Read the model definition and answer for the solid it produces. Units are mm, in the model's axes. A direction names the side the tool comes from. Give positions to 0.01 mm unless a question says otherwise; leave off trailing zeros. Order: outer loops, then holes, each group sorted by start corner. A loop starts at its lowest first (then second) coordinate and runs counter-clockwise, first axis right, second up. Notation, with made-up numbers: (58, -29) - (117, -29) arc R20 cw to (117, -24) - close; hole circle Ø2 at (42, 47). An arc over 180 degrees is marked (long way). Use a Markdown table: item, result. Add a question column.
1. A cutting plane is placed at A-A on y = -5. Determine the outline of the cut face in (x, z).
2. Which of the six approach directions +Z, -Z, +X, -X, +Y, -Y give full straight-line access (tool end or side, diameter ignored) to faces 1 (the flat face through (-51, -19, 0)), 2 (the flat face through (-70, -35, 5))?
3. Consider L1, parallel to Z at x = -64.5, y = -24.5; L2, parallel to Z at x = -42, y = -24.5; L3, parallel to X at y = -41.5, z = -0.5. Determine where each line is inside the solid, lowest interval first.
4. A flat-ended cylindrical pin translates along its axis: P1, Ø6, axis at y = -58, z = 7.5, coming from the +X side. Find the tip coordinate at first contact, or state that the pin passes through.
```python
from build123d import *

# Parameters (mm, degrees)
SKETCH_W    = 70
SKETCH_H    = 70
PAD_DEPTH   = 10
SKETCH004_W = 20
SKETCH004_H = 20
SKETCH003_W = 30
SKETCH003_H = 30
FILLET_R    = 2


with BuildPart() as part:
    # Sketch → Pad (new body)
    with BuildSketch(Plane.XY):
        with Locations((-35, -35)):
            Rectangle(SKETCH_W, SKETCH_H)
    extrude(amount=PAD_DEPTH)

    # Sketch004 (on DatumPlane) → AdditiveLoft section 0
    with BuildSketch(Plane.XY.offset(-10)):
        with Locations((-35, -35)):
            Rectangle(SKETCH004_W, SKETCH004_H)
    # Sketch003 (on Face5 of Pad) → AdditiveLoft section 1
    with BuildSketch(Plane(origin=(0, 0, 0), x_dir=(1, 0, 0), z_dir=(0, 0, -1))):
        with Locations((-35, 35)):
            Rectangle(SKETCH003_W, SKETCH003_H)
    loft()

    # Fillet
    fillet_edges = [part.edges().sort_by_distance(p)[0] for p in [
        (-45, -35, -10),
        (-47.5, -22.5, -5),
        (-50, -35, 0),
        (-47.5, -47.5, -5),
        (-35, -25, -10),
        (-22.5, -22.5, -5),
        (-35, -20, 0),
        (-25, -35, -10),
        (-22.5, -47.5, -5),
        (-20, -35, 0),
        (-35, -45, -10),
        (-35, -50, 0),
    ]]
    fillet(fillet_edges, radius=FILLET_R)


solid = part.part
```
Output values:
| question | item | result |
|---|---|---|
| 1 | outline | (-70, 0) - (0, 0) - (0, 10) - (-70, 10) - close |
| 2 | face 1 | -Z |
| 2 | face 2 | +Z, -Z, -X, +Y, -Y |
| 3 | L1 | 0 to 10 |
| 3 | L2 | -8.99 to 10 |
| 3 | L3 | -49.91 to -20.09 |
| 4 | P1 | x = 0 |
